Model file for the job. Use its own axes, mm. Give positions to 0.01 mm unless a question says otherwise; leave off trailing zeros. Write each loop counter-clockwise with the first axis right and the second up, starting at its lowest first coordinate (ties: lowest second). Pieces come first, ordered by that corner, then holes. Notation, with made-up numbers: M 39.25,-34 L 73.25,-34 A31 ccw 73.25,-2 Z; hole C -26.75,83 d4. An arc over 180 degrees is marked long. Answer as a JSON object with one key per item and string values. Group by question number.
```python
from build123d import *

# Parameters (mm, degrees)
BOSS_EXTRUDE3_DEPTH = 10
LPATTERN1_COUNT     = 4
LPATTERN1_PITCH     = 2
SKETCH3_R           = 2.375
CUT_EXTRUDE1_DEPTH  = 14.747727085
FILLET1_R           = 0.2


with BuildPart() as part:
    # Sketch2 → Boss-Extrude3 (new body)
    with BuildSketch(Plane.XY):
        Polygon((-5, 1), (-1.183578012, 0), (0, 0.310127658), (-2.632843976, 1), (0, 1.689872342), (-1.183578012, 2), align=None)
        Polygon((0, 0.310127658), (1.183578012, 0), (5, 1), (1.183578012, 2), (0, 1.689872342), (2.632843976, 1), align=None)
        Polygon((1.183578012, 2), (-1.183578012, 2), (0, 1.689872342), align=None)
        Polygon((0, 0.310127658), (-1.183578012, 0), (1.183578012, 0), align=None)
    boss_extrude3 = extrude(amount=BOSS_EXTRUDE3_DEPTH)

    # LPattern1: Boss-Extrude3 ×4
    with Locations(*[(0, i * LPATTERN1_PITCH, 0) for i in range(1, LPATTERN1_COUNT)]):
        add(boss_extrude3)

    # Sketch3 → Cut-Extrude1 (cut, through all)
    with BuildSketch(Plane.XZ):
        with Locations(Location((0, 5, 0), (0, 0, 270))):
            Circle(SKETCH3_R)
    extrude(amount=-CUT_EXTRUDE1_DEPTH, mode=Mode.SUBTRACT)

    # Fillet1
    fillet1_edges = [part.edges().sort_by_distance(p)[0] for p in [
        (5, 1, 5),
        (-5, 1, 5),
        (5, 3, 5),
        (-5, 3, 5),
        (5, 5, 5),
        (-5, 5, 5),
        (5, 7, 5),
        (-5, 7, 5),
    ]]
    fillet(fillet1_edges, radius=FILLET1_R)


solid = part.part
```
Q1. Drop flat-ended pins along their axis: P1, Ø4, axis at x = 0, z = 5, coming from the +Y side; P2, Ø1.5, axis at y = 4.5, z = 5.5, coming from the +X side. Give the stop position or say it passes through.
Q2. Slice it at B-B, the plane z = 0.5. Count the separate pieces of the cut face and the enclosed holes in it, then the cut area to 3 significant figures.
Q3. Wall check: L1, parallel to Y at x = 3.75, z = 1; L2, parallel to Z at x = 0, y = 4.2 (3 decimals); L3, parallel to Y at x = 3.25, z = 6. Give the ranges that are in metal, low to high.
Q4. Two-plate mould, pull along Z, no slides. Class faces 1 (the flat face through (0, 4, 0)), 2 (the flat face through (0, 8, 9)), 3 (the cylindrical face through (0.713, 1.987, 2.735)): +Z half, -Z half, draft (parallel to the pull), parting line (faces both ways), or undercut.
Q5. Slice it at A-A, the plane y = 6.5. Write the cut outline in (x, z) (3 decimals), then the cut area to 3 significant figures.
Solved:
{
 "1": {"P1": "passes through", "P2": "stops at x = 4.41"},
 "2": {"separate pieces": "1", "enclosed holes": "4", "area": "34.1 mm²"},
 "3": {"L1": "y = 0.67 to 1.33, 2.67 to 3.33, 4.67 to 5.33, 6.67 to 7.33", "L2": "z = 0 to 2.625, 7.375 to 10", "L3": "y = 0.54 to 1.46, 2.54 to 3.46, 4.54 to 5.46, 6.54 to 7.46"},
 "4": {"face 1": "-Z half", "face 2": "draft", "face 3": "undercut"},
 "5": {"outline": "M -3.092,0 L -0.725,0 L -0.725,2.738 A2.375 cw -0.725,7.262 L -0.725,10 L -3.092,10 Z; M 0.725,0 L 3.092,0 L 3.092,10 L 0.725,10 L 0.725,7.262 A2.375 cw 0.725,2.738 Z", "area": "36.4 mm²"}
}
